Work out the finished part from the listing and answer in its coordinate system (mm). Face numbers are marked on the shaded views. A direction names the side the tool comes from. Round coordinates to 2 decimals unless told otherwise and drop trailing zeros. Order: outer loops, then holes, each group sorted by start corner. A loop starts at its lowest first (then second) coordinate and runs counter-clockwise, first axis right, second up. Notation, with made-up numbers: (37, -32) - (53, -32) arc R21 ccw to (53, -25) - close; hole circle Ø2 at (-18, 60.5). An arc over 180 degrees is marked (long way). Answer in a Markdown table with one row per item.
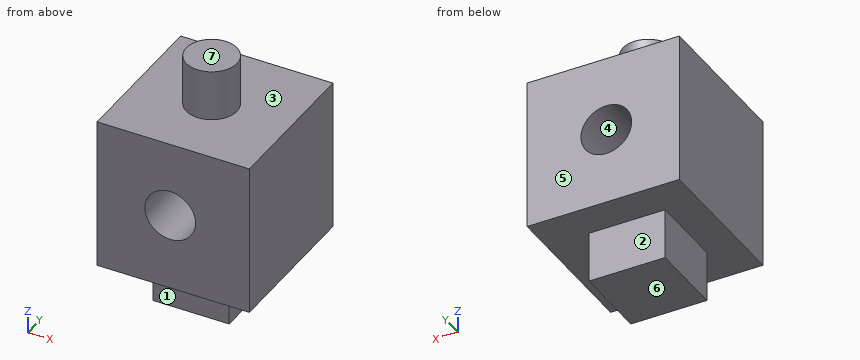
from build123d import *

# Parameters (mm, degrees)
F0_W     = 76.2
F0_H     = 76.2
F1_DEPTH = 76.2
F2_R     = 12.7
F3_DEPTH = 76.2
F4_R     = 12.7
F5_DEPTH = 25.4
F6_W     = 38.1
F6_H     = 38.1
F7_DEPTH = 25.4


with BuildPart() as f1:
    # F0 (on Top) → F1 (new body)
    with BuildSketch(Plane.XY):
        with Locations((-38.1, 38.1)):
            Rectangle(F0_W, F0_H)
    extrude(amount=F1_DEPTH)

    # F2 (on face) → F3 (cut)
    with BuildSketch(Plane.XZ):
        with Locations((-39.623093, 38.477365)):
            Circle(F2_R)
    extrude(amount=-F3_DEPTH, mode=Mode.SUBTRACT)

    # F4 (on face) → F5 (join)
    with BuildSketch(Plane.XY.offset(76.2)):
        with Locations((-39.050225, 36.758773)):
            Circle(F4_R)
    extrude(amount=F5_DEPTH)

    # F6 (on face) → F7 (join)
    with BuildSketch(Plane(origin=(0, 0, 0), x_dir=(1, 0, 0), z_dir=(0, 0, -1))):
        with Locations((-40.341444, -39.477604)):
            Rectangle(F6_W, F6_H)
    extrude(amount=F7_DEPTH)


solid = f1.part
1) Find section D-D, the plane z = -7. Give the vertices of the cut face in (x, y).
Filled in:
| item | result |
|---|---|
| outline | (-59.39, 20.43) - (-21.29, 20.43) - (-21.29, 58.53) - (-59.39, 58.53) - close |
2) Which of the six approach directions +Z, -Z, +X, -X, +Y, -Y give full straight-line access (tool end or side, diameter ignored) to the marked faces 1, 2 and 3?
Filled in:
| item | result |
|---|---|
| face 1 | -Z, +X, -X, -Y |
| face 2 | -Z, +X, -X, +Y |
| face 3 | +Z |
3) Find section A-A, the plane x = -39. Give the vertices of the cut face in (y, z).
Filled in:
| item | result |
|---|---|
| outline | (0, 0) - (20.43, 0) - (20.43, -25.4) - (58.53, -25.4) - (58.53, 0) - (76.2, 0) - (76.2, 25.79) - (0, 25.79) - close; (0, 51.16) - (76.2, 51.16) - (76.2, 76.2) - (49.46, 76.2) - (49.46, 101.6) - (24.06, 101.6) - (24.06, 76.2) - (0, 76.2) - close |
4) Find the intervals of material crossed by probe 1 along X at (y, z) = (21, -9.5); probe 2 along Z at (x, y) = (-22, 42); probe 3 along Z at (x, y) = (-33, 40.5), in increasing order. Write a range as from..to.
Filled in:
| item | result |
|---|---|
| probe 1 | x = -59.39..-21.29 |
| probe 2 | z = -25.4..76.2 |
| probe 3 | z = -25.4..27.64, 49.31..101.6 |
5) Find section C-C, the plane y = 31. Give the vertices of the cut face in (x, z), then the cut area to 3 significant figures.
Filled in:
| item | result |
|---|---|
| outline | (-76.2, 0) - (-59.39, 0) - (-59.39, -25.4) - (-21.29, -25.4) - (-21.29, 0) - (0, 0) - (0, 76.2) - (-27.73, 76.2) - (-27.73, 101.6) - (-50.37, 101.6) - (-50.37, 76.2) - (-76.2, 76.2) - close; hole circle Ø25.4 at (-39.62, 38.48) |
| area | 6,840 mm^2 |
6) Each of these flat-tipped pins is pushed along its axis until it touches: pin 1 (7.5 mm diameter, centred on y = 47, z = -14, fed in from +X); pin 2 (20.5 mm diameter, centred on x = -49, z = -14, fed in from +Y); pin 3 (7.5 mm diameter, centred on x = -47, z = -14.5, fed in from -Y). Where does it stop, or does it pass through?
Filled in:
| item | result |
|---|---|
| pin 1 | stops at x = -21.29 |
| pin 2 | stops at y = 58.53 |
| pin 3 | stops at y = 20.43 |
7) The mould has two halves that part along Z. Classify the marked faces 4, 5, 6 and 7: released by +Z, released by -Z, zero draft, split by the parting line, or undercut.
Filled in:
| item | result |
|---|---|
| face 4 | undercut |
| face 5 | zero draft |
| face 6 | released by -Z |
| face 7 | released by +Z |
8) Find section B-B, the plane z = 40. Give the vertices of the cut face in (x, y), then the cut area to 3 significant figures.
Filled in:
| item | result |
|---|---|
| outline | (-76.2, 0) - (-52.23, 0) - (-52.23, 76.2) - (-76.2, 76.2) - close; (-27.01, 0) - (0, 0) - (0, 76.2) - (-27.01, 76.2) - close |
| area | 3,880 mm^2 |
